```python
from build123d import *

# Parameters (mm, degrees)
SKETCH1_W           = 520
SKETCH1_H           = 380
BOSS_EXTRUDE1_DEPTH = 2.778125
SKETCH2_W           = 220
SKETCH2_H           = 190
CUT_EXTRUDE1_DEPTH  = 2.778125
SKETCH3_W           = 100
SKETCH3_H           = 220
CUT_EXTRUDE2_DEPTH  = 2.778125
FILLET2_R           = 60
FILLET3_R           = 60
SKETCH4_R           = 21
CUT_EXTRUDE3_DEPTH  = 2.778125


with BuildPart() as part:
    # Sketch1 → Boss-Extrude1 (new body)
    with BuildSketch(Plane.XY):
        with Locations((-200, 190)):
            Rectangle(SKETCH1_W, SKETCH1_H)
    extrude(amount=BOSS_EXTRUDE1_DEPTH)

    # Sketch2 → Cut-Extrude1 (cut)
    with BuildSketch(Plane.XY.offset(2.778125)):
        with Locations((-50, 285)):
            Rectangle(SKETCH2_W, SKETCH2_H)
    extrude(amount=-CUT_EXTRUDE1_DEPTH, mode=Mode.SUBTRACT)

    # Sketch3 → Cut-Extrude2 (cut)
    with BuildSketch(Plane.XY.offset(2.778125)):
        with Locations((-410, 110)):
            Rectangle(SKETCH3_W, SKETCH3_H)
    extrude(amount=-CUT_EXTRUDE2_DEPTH, mode=Mode.SUBTRACT)

    # Fillet2
    fillet2_edges = [part.edges().sort_by_distance(p)[0] for p in [
        (-460, 220, 1.3890625),
        (-460, 380, 1.3890625),
    ]]
    fillet(fillet2_edges, radius=FILLET2_R)

    # Fillet3
    fillet3_edges = [part.edges().sort_by_distance(p)[0] for p in [
        (60, 190, 1.3890625),
        (-160, 380, 1.3890625),
        (-360, 0, 1.3890625),
        (60, 0, 1.3890625),
    ]]
    fillet(fillet3_edges, radius=FILLET3_R)

    # Sketch4 → Cut-Extrude3 (cut)
    with BuildSketch(Plane.XY.offset(2.778125)):
        with Locations((-395.138918322, 295)):
            Circle(SKETCH4_R)
        with Locations((-245.138918322, 295)):
            Circle(SKETCH4_R)
        with Locations((-245.138918322, 95)):
            Circle(SKETCH4_R)
        with Locations((-45.138918322, 95)):
            Circle(SKETCH4_R)
    extrude(amount=-CUT_EXTRUDE3_DEPTH, mode=Mode.SUBTRACT)


solid = part.part
```
Verification items for the finished model (mm, model axes). Round coordinates to 2 decimals unless told otherwise and drop trailing zeros. Order: outer loops, then holes, each group sorted by start corner. A loop starts at its lowest first (then second) coordinate and runs counter-clockwise, first axis right, second up. Notation, with made-up numbers: (-21, 76.25) - (16, 76.25) arc R24 ccw to (16, 114.25) - close; hole circle Ø2 at (47.5, 40). An arc over 180 degrees is marked (long way). Use CSV: the item, a comma, the result in double quotes. Start each with the question number.
1) Section check C-C, the plane y = 200. Record the cut outline in (x, z).
2) Thickness scan on L1, parallel to Y at x = -245, z = 1.45; L2, parallel to Y at x = -248.5, z = 0.4; L3, parallel to X at y = 312, z = 1.6. Record the ranges inside material, lowest first.
3) Mould release check, pull along X, two halves, no side actions. Record for faces 1 (the cylindrical face through (-225.74, 286.96, 1.41)), 2 (the cylindrical face through (-442.89, 238.04, 1.37)), 3 (the cylindrical face through (-49.7, 74.5, 1.4)), 4 (the flat face through (-204, 193, 2.778)): +X half, -X half, draft (parallel to the pull), parting line (faces both ways), or undercut.
4) Section check B-B, the plane z = 1.25. Record the cut outline in (x, y).
5) Section check A-A, the plane y = 95. Record the cut outline in (x, z), plus the area to 3 significant figures.
6) Section check D-D, the plane y = 295. Record the cut outline in (x, z).
7) Go/stop test with flat-tipped pins: P1, Ø1.4, axis at x = -77.5, z = 1.5, coming from the +Y side; P2, Ø1.4, axis at y = 175, z = 1, coming from the -X side; P3, Ø0.8, axis at y = 238, z = 1.5, coming from the +X side; P4, Ø8, axis at x = -228.5, y = 77.5, coming from the -Z side. Record where each tip stops, or that it passes through.
Answers:
1,outline,"(-360, 0) - (-160, 0) - (-160, 2.78) - (-360, 2.78) - close"
2,L1,"y = 0 to 74, 116 to 274, 316 to 380"
2,L2,"y = 0 to 74.27, 115.73 to 274.27, 315.73 to 380"
2,L3,"x = -460 to -407.47, -382.81 to -257.47, -232.81 to -160"
3,face 1,"undercut"
3,face 2,"-X half"
3,face 3,"undercut"
3,face 4,"draft"
4,outline,"(-460, 280) arc R60 ccw to (-400, 220) - (-360, 220) - (-360, 60) arc R60 ccw to (-300, 0) - (0, 0) arc R60 ccw to (60, 60) - (60, 130) arc R60 ccw to (0, 190) - (-160, 190) - (-160, 320) arc R60 ccw to (-220, 380) - (-400, 380) arc R60 ccw to (-460, 320) - close; hole circle Ø42 at (-395.14, 295); hole circle Ø42 at (-245.14, 95); hole circle Ø42 at (-245.14, 295); hole circle Ø42 at (-45.14, 95)"
5,outline,"(-360, 0) - (-266.14, 0) - (-266.14, 2.78) - (-360, 2.78) - close; (-224.14, 0) - (-66.14, 0) - (-66.14, 2.78) - (-224.14, 2.78) - close; (-24.14, 0) - (60, 0) - (60, 2.78) - (-24.14, 2.78) - close"
5,area,"933 mm²"
6,outline,"(-460, 0) - (-416.14, 0) - (-416.14, 2.78) - (-460, 2.78) - close; (-374.14, 0) - (-266.14, 0) - (-266.14, 2.78) - (-374.14, 2.78) - close; (-224.14, 0) - (-160, 0) - (-160, 2.78) - (-224.14, 2.78) - close"
7,P1,"stops at y = 190"
7,P2,"stops at x = -360"
7,P3,"stops at x = -160"
7,P4,"stops at z = 0"
